from build123d import *

# Parameters (mm, degrees)
ESBO_O1_R                = 1.5
ESBO_O1_R_2              = 3.5
ESBO_O1_R_3              = 2.5
RESSALTO_EXTRUS_O2_DEPTH = 6
FILETE1_R                = 15
ESBO_O2_R                = 3
CORTE_EXTRUS_O1_DEPTH    = 10


with BuildPart() as part:
    # Esboço1 → Ressalto-extrusão2 (new body)
    with BuildSketch(Plane.XY):
        Polygon((0, 0), (0, 220), (50, 220), (100, 0), align=None)
        with Locations((17, 210)):
            Circle(ESBO_O1_R, mode=Mode.SUBTRACT)
        with Locations(Location((33, 210, 0), (0, 0, 180))):
            Circle(ESBO_O1_R, mode=Mode.SUBTRACT)
        with Locations((33, 190)):
            Circle(ESBO_O1_R, mode=Mode.SUBTRACT)
        with Locations(Location((17, 190, 0), (0, 0, 180))):
            Circle(ESBO_O1_R, mode=Mode.SUBTRACT)
        with Locations((25, 200)):
            Circle(ESBO_O1_R_2, mode=Mode.SUBTRACT)
        with Locations((10, 30)):
            Circle(ESBO_O1_R_3, mode=Mode.SUBTRACT)
        with BuildLine():
            Line((20, 95), (20, 66))
            ThreePointArc((20, 66), (20.878679656, 63.878679656), (23, 63))
            Line((23, 63), (61.413470366, 63))
            ThreePointArc((61.413470366, 63), (63.75810146, 64.128448496), (64.338868934, 66.664863311))
            Line((64.338868934, 66.664863311), (57.747959843, 95.664863311))
            ThreePointArc((57.747959843, 95.664863311), (56.69411278, 97.344631094), (54.822561275, 98))
            Line((54.822561275, 98), (23, 98))
            ThreePointArc((23, 98), (20.878679656, 97.121320344), (20, 95))
        make_face(mode=Mode.SUBTRACT)
        with BuildLine():
            Line((20, 40), (20, 23))
            ThreePointArc((20, 23), (20.878679656, 20.878679656), (23, 20))
            Line((23, 20), (71.186197639, 20))
            ThreePointArc((71.186197639, 20), (73.530828733, 21.128448496), (74.111596206, 23.664863311))
            Line((74.111596206, 23.664863311), (70.247959843, 40.664863311))
            ThreePointArc((70.247959843, 40.664863311), (69.19411278, 42.344631094), (67.322561275, 43))
            Line((67.322561275, 43), (23, 43))
            ThreePointArc((23, 43), (20.878679656, 42.121320344), (20, 40))
        make_face(mode=Mode.SUBTRACT)
    extrude(amount=RESSALTO_EXTRUS_O2_DEPTH)

    # Filete1
    filete1_edges = [part.edges().sort_by_distance(p)[0] for p in [
        (0, 220, 3),
        (50, 220, 3),
    ]]
    fillet(filete1_edges, radius=FILETE1_R)

    # Esboço2 → Corte-extrusão1 (cut)
    with BuildSketch(Plane(origin=(0, 0, 0), x_dir=(-1, 0, 0), z_dir=(0, 0, -1))):
        with Locations((-90.096252795, 14.5)):
            Circle(ESBO_O2_R)
    extrude(amount=-CORTE_EXTRUS_O1_DEPTH, mode=Mode.SUBTRACT)


solid = part.part
CAD build for the part. Positions are in the model's coordinates, mm. A direction names the side the tool comes from. Give positions to 0.01 mm unless a question says otherwise; leave off trailing zeros. Order: outer loops, then holes, each group sorted by start corner. A loop starts at its lowest first (then second) coordinate and runs counter-clockwise, first axis right, second up. Notation, with made-up numbers: (30.25, -20) - (89.25, -20) arc R20 ccw to (89.25, 2) - close; hole circle Ø1 at (25, 84.5). An arc over 180 degrees is marked (long way). Write each question's results on one line, items separated by ' | '.
1. Pin check, flat tips, straight feed: pin 1 (3 mm diameter, centred on x = 44, z = 4, fed in from +Y); pin 2 (1.8 mm diameter, centred on y = 76.5, z = 3.5, fed in from +X); pin 3 (2.5 mm diameter, centred on x = 33, y = 210, fed in from -Z). Stop position of each tip, or through.
Calculated:
pin 1: stops at y = 219.32 | pin 2: stops at x = 82.82 | pin 3: passes through
2. Pull direction Y, two halves, no side cores. Call faces 3 (the face through (24.241, 196.583, 2.958)), 4 (the face through (4.28, 215.49, 3.04)), 5 (the face through (51, 0, 3)), 6 (the face through (72.207, 32.046, 2.958)): released by +Y, released by -Y, zero draft, split by the parting line, or undercut.
Calculated:
face 3: undercut | face 4: released by +Y | face 5: released by -Y | face 6: undercut
3. 3-axis set-ups, long thin cutter, end or side, ignore diameter. For faces 1 (the face through (20, 32, 3)), 2 (the face through (26, 220, 3)): which of +Z, -Z, +X, -X, +Y, -Y reach the whole face in a straight line?
Calculated:
face 1: +Z, -Z | face 2: +Z, -Z, +X, -X, +Y
4. Saw through at D-D on x = 89.5. List the corners of the cut face in (y, z), and give its area (3 significant figures).
Calculated:
outline: (0, 0) - (11.56, 0) - (11.56, 6) - (0, 6) - close; (17.44, 0) - (46.2, 0) - (46.2, 6) - (17.44, 6) - close | area: 242 mm2
5. Saw through at A-A on x = 45. List the corners of the cut face in (y, z).
Calculated:
outline: (0, 0) - (20, 0) - (20, 6) - (0, 6) - close; (43, 0) - (63, 0) - (63, 6) - (43, 6) - close; (98, 0) - (218.28, 0) - (218.28, 6) - (98, 6) - close
6. Probe L1, parallel to Y at x = 25, z = 4.55; L2, parallel to Y at x = 17, z = 4.1; L3, parallel to Y at x = 33, z = 3.4. List the from-to ranges inside material, lowest first. Write a range as from..to.
Calculated:
L1: y = 0..20, 43..63, 98..196.5, 203.5..220 | L2: y = 0..188.5, 191.5..208.5, 211.5..220 | L3: y = 0..20, 43..63, 98..188.5, 191.5..208.5, 211.5..220
7. Saw through at B-B on y = 76. List the corners of the cut face in (x, z).
Calculated:
outline: (0, 0) - (20, 0) - (20, 6) - (0, 6) - close; (62.22, 0) - (82.73, 0) - (82.73, 6) - (62.22, 6) - close
8. Saw through at C-C on z = 4.3. Count the separate pieces of the cut face and the enclosed holes in it, and give its area (3 significant figures).
Calculated:
separate pieces: 1 | enclosed holes: 9 | area: 13,700 mm2
